```python
from build123d import *

# Parameters (mm, degrees)
SKETCH20_W            = 172.0559932
SKETCH20_H            = 108.5559932
BOSS_EXTRUDE5_DEPTH   = 1.699999902
BOSS_EXTRUDE6_DEPTH   = 1.7
FILLET3_R             = 2.54
F_4_40_TAPPED_HOLE3_D = 2.2606


with BuildPart() as part:
    # Sketch20 → Boss-Extrude5 (new body)
    with BuildSketch(Plane(origin=(0, 0, 0), x_dir=(1, 0, 0), z_dir=(0, 1, 0))):
        with Locations((84.0279966, 74.0579966)):
            Rectangle(SKETCH20_W, SKETCH20_H)
    extrude(amount=-BOSS_EXTRUDE5_DEPTH)

    # Sketch20<3> → Boss-Extrude6 (add)
    with BuildSketch(Plane(origin=(0, 0, 0), x_dir=(1, 0, 0), z_dir=(0, 1, 0))):
        with BuildLine():
            Line((2.572, 21.812), (165.4839932, 21.812))
            ThreePointArc((165.4839932, 21.812), (166.227941976, 23.608051224), (168.0239932, 24.352))
            Line((168.0239932, 24.352), (168.0239932, 123.7639932))
            ThreePointArc((168.0239932, 123.7639932), (166.227941976, 124.507941976), (165.4839932, 126.3039932))
            Line((165.4839932, 126.3039932), (2.572, 126.3039932))
            ThreePointArc((2.572, 126.3039932), (1.828051224, 124.507941976), (0.032, 123.7639932))
            Line((0.032, 123.7639932), (0.032, 24.352))
            ThreePointArc((0.032, 24.352), (1.828051224, 23.608051224), (2.572, 21.812))
        make_face()
        with BuildLine():
            Line((3.624102448, 23.082), (164.431890752, 23.082))
            ThreePointArc((164.431890752, 23.082), (165.329916364, 24.506076836), (166.7539932, 25.404102448))
            Line((166.7539932, 25.404102448), (166.7539932, 122.711890752))
            ThreePointArc((166.7539932, 122.711890752), (165.329916364, 123.609916364), (164.431890752, 125.0339932))
            Line((164.431890752, 125.0339932), (3.624102448, 125.0339932))
            ThreePointArc((3.624102448, 125.0339932), (2.726076836, 123.609916364), (1.302, 122.711890752))
            Line((1.302, 122.711890752), (1.302, 25.404102448))
            ThreePointArc((1.302, 25.404102448), (2.726076836, 24.506076836), (3.624102448, 23.082))
        make_face(mode=Mode.SUBTRACT)
    extrude(amount=BOSS_EXTRUDE6_DEPTH)

    # Fillet3
    fillet3_edges = [part.edges().sort_by_distance(p)[0] for p in [
        (-2, -0.849999951, -128.3359932),
        (-2, -0.849999951, -19.78),
        (170.0559932, -0.849999951, -19.78),
        (170.0559932, -0.849999951, -128.3359932),
    ]]
    fillet(fillet3_edges, radius=FILLET3_R)

    # #4-40 Tapped Hole3 (through all)
    with Locations(Plane(origin=(0, 0, 0), x_dir=(1, 0, 0), z_dir=(0, 1, 0))):
        with Locations((0.032, 21.812), (168.0239932, 21.812), (168.0239932, 126.3039932), (0.032, 126.3039932)):
            Hole(F_4_40_TAPPED_HOLE3_D / 2)


solid = part.part
```
Work out the finished part from the listing and answer in its coordinate system (mm). Give positions to 0.01 mm unless a question says otherwise; leave off trailing zeros. Write each loop counter-clockwise with the first axis right and the second up, starting at its lowest first coordinate (ties: lowest second). Pieces come first, ordered by that corner, then holes.
(1) The part is cut by section B-B on z = -45. Write down the section's boundary in (x, y).
Final values:
outline: (-2, -1.7) - (170.06, -1.7) - (170.06, 0) - (168.02, 0) - (168.02, 1.7) - (166.75, 1.7) - (166.75, 0) - (1.3, 0) - (1.3, 1.7) - (0.03, 1.7) - (0.03, 0) - (-2, 0) - close
(2) Straight lines are drawn through the part: line 1 (Z direction, x = 49.5, y = 1.4); line 2 (Y direction, x = 150.5, z = -57); line 3 (X direction, y = 0.9, z = -107.5). For each, find the intervals that lie inside material, in ascending order.
Final values:
line 1: z = -126.3 to -125.03, -23.08 to -21.81
line 2: y = -1.7 to 0
line 3: x = 0.03 to 1.3, 166.75 to 168.02
(3) The part is cut by section A-A on y = 1.15. Write down the section's boundary in (x, z).
Final values:
outline: (0.03, -123.76) arc R2.54 cw to (2.57, -126.3) - (165.48, -126.3) arc R2.54 cw to (168.02, -123.76) - (168.02, -24.35) arc R2.54 cw to (165.48, -21.81) - (2.57, -21.81) arc R2.54 cw to (0.03, -24.35) - close; hole (1.3, -122.71) arc R3.81 cw to (3.62, -125.03) - (164.43, -125.03) arc R3.81 cw to (166.75, -122.71) - (166.75, -25.4) arc R3.81 cw to (164.43, -23.08) - (3.62, -23.08) arc R3.81 cw to (1.3, -25.4) - close
(4) Flat-ended cylindrical pins translate along their axes: pin 1 Ø1.9 at (y, z) = (1, -79.5) entering from +X; pin 2 Ø1.5 at (y, z) = (1, -52.5) entering from -X; pin 3 Ø3.5 at (x, z) = (168.02, -126.3) entering from -Y; pin 4 Ø1.8 at (x, z) = (168.02, -21.81) entering from -Y. Find the tip coordinate at first contact, or state that the pin passes through.
Final values:
pin 1: stops at x = 168.02
pin 2: stops at x = 0.03
pin 3: stops at y = -1.7
pin 4: passes through
(5) The mould has two halves that part along X. Classify faces 1 (the flat face through (90, 0, -127)), 2 (the flat face through (83, 0, -75)): pulls with the +X half, pulls with the -X half, needs draft (parallel to the pull), parting line crosses it, or undercut.
Final values:
face 1: needs draft
face 2: undercut
(6) The part is cut by section C-C on x = 44. Write down the section's boundary in (y, z).
Final values:
outline: (-1.7, -128.34) - (0, -128.34) - (0, -126.3) - (1.7, -126.3) - (1.7, -125.03) - (0, -125.03) - (0, -23.08) - (1.7, -23.08) - (1.7, -21.81) - (0, -21.81) - (0, -19.78) - (-1.7, -19.78) - close
